Build history of the part. All positions in model axes, mm. A direction names the side the tool comes from. Round coordinates to 2 decimals unless told otherwise and drop trailing zeros. Write each loop counter-clockwise with the first axis right and the second up, starting at its lowest first coordinate (ties: lowest second). Pieces come first, ordered by that corner, then holes. Notation, with made-up numbers: (57, 45.5) -> (103, 45.5) arc R19 cw to (103, 58.5) -> close; hole circle Ø6 at (-3, -17). An arc over 180 degrees is marked (long way). Answer in a Markdown table with one row per item.
Autodesk Inventor part; units mm, degrees
ref_plane "YZ Plane" through (0, 0, 0) normal (1, 0, 0) x (0, 1, 0)
ref_plane "XZ Plane" through (0, 0, 0) normal (0, 1, 0) x (-1, 0, 0)
ref_plane "XY Plane" through (0, 0, 0) normal (0, 0, 1) x (1, 0, 0)
sketch "Skizze1" plane through (0, 0, 0) normal (0, 0, 1) x (1, 0, 0)
  line L0 (0, 0) -> (43.18, 0)
  line L1 (43.18, 0) -> (43.18, 20)
  line L2 (43.18, 20) -> (0, 20)
  line L3 (0, 20) -> (0, 0)
  circle A0 centre (2.54, 2.761) radius 1.651
  circle A1 centre (40.64, 17.239) radius 1.651
  line L4 (21.59, 20) -> (21.59, 0) construction
  line L5 (2.54, 2.761) -> (40.64, 2.761) construction
  line L6 (40.64, 2.761) -> (40.64, 17.239) construction
  line L7 (40.64, 17.239) -> (2.54, 17.239) construction
  line L8 (2.54, 17.239) -> (2.54, 2.761) construction
  line L9 (0, 10) -> (43.18, 10) construction
  line L10 (21.965, 2.2486) -> (21.215, 2.2486)
  line L11 (21.215, 2.2486) -> (21.215, 1.4986)
  line L12 (21.215, 1.4986) -> (21.965, 1.4986)
  line L13 (21.965, 1.4986) -> (21.965, 2.2486)
  line L14 (24.715, 2.2486) -> (23.965, 2.2486)
  line L15 (24.715, 1.4986) -> (24.715, 2.2486)
  line L16 (23.965, 1.4986) -> (24.715, 1.4986)
  line L17 (23.965, 2.2486) -> (23.965, 1.4986)
  line L18 (27.465, 2.2486) -> (26.715, 2.2486)
  line L19 (27.465, 1.4986) -> (27.465, 2.2486)
  line L20 (26.715, 1.4986) -> (27.465, 1.4986)
  line L21 (26.715, 2.2486) -> (26.715, 1.4986)
  line L22 (19.215, 2.2486) -> (18.465, 2.2486)
  line L23 (19.215, 1.4986) -> (19.215, 2.2486)
  line L24 (18.465, 1.4986) -> (19.215, 1.4986)
  line L25 (18.465, 2.2486) -> (18.465, 1.4986)
  line L26 (21.965, 2.2486) -> (21.215, 2.2486)
  line L27 (21.965, 1.4986) -> (21.965, 2.2486)
  line L28 (21.215, 1.4986) -> (21.965, 1.4986)
  line L29 (21.215, 2.2486) -> (21.215, 1.4986)
  line L30 (24.715, 2.2486) -> (23.965, 2.2486)
  line L31 (24.715, 1.4986) -> (24.715, 2.2486)
  line L32 (23.965, 1.4986) -> (24.715, 1.4986)
  line L33 (23.965, 2.2486) -> (23.965, 1.4986)
  line L34 (16.465, 2.2486) -> (15.715, 2.2486)
  line L35 (16.465, 1.4986) -> (16.465, 2.2486)
  line L36 (15.715, 1.4986) -> (16.465, 1.4986)
  line L37 (15.715, 2.2486) -> (15.715, 1.4986)
  line L38 (19.215, 2.2486) -> (18.465, 2.2486)
  line L39 (19.215, 1.4986) -> (19.215, 2.2486)
  line L40 (18.465, 1.4986) -> (19.215, 1.4986)
  line L41 (18.465, 2.2486) -> (18.465, 1.4986)
  line L42 (21.965, 2.2486) -> (21.215, 2.2486)
  line L43 (21.965, 1.4986) -> (21.965, 2.2486)
  line L44 (21.215, 1.4986) -> (21.965, 1.4986)
  line L45 (21.215, 2.2486) -> (21.215, 1.4986)
  point P0 (21.59, 17.239)
  point P1 (40.64, 10)
  point P2 (21.59, 2.2486)
  point P3 (24.34, 2.2486)
  point P4 (27.09, 2.2486)
  point P5 (18.84, 2.2486)
  point P6 (21.59, 2.2486)
  point P7 (24.34, 2.2486)
  point P8 (16.09, 2.2486)
  point P9 (18.84, 2.2486)
  point P10 (21.59, 2.2486)
  dimension "d0" = 43.18
  dimension "d1" = 20
  dimension "d2" = 3.302
  dimension "d4" = 38.1
  dimension "d5" = 14.478
  dimension "d26" = 1.4986
  dimension "d27" = 0.75
  dimension "d30" = 2.75
  dimension "d33" = 2.75
extrude "Extrusion1" add sketch "Skizze1" against normal blind 1.524
sketch "Skizze2" plane through (0, 0, 0) normal (0, 0, 1) x (1, 0, 0)
  circle A0 centre (10.1127, 10) radius 8.128
  circle A1 centre (33.0673, 10) radius 8.128
  line L0 (0, 0) -> (0, 20) construction
  line L1 (0, 10) -> (43.18, 10) construction
  line L2 (43.18, 0) -> (43.18, 20) construction
  line L3 (10.1127, 10) -> (33.0673, 10) construction
  point P0 (21.59, 10)
  dimension "d19" = 16.256
extrude "Extrusion2" add sketch "Skizze2" along normal blind 12.7
fillet "Rundung1" radius 1 2 edges at (24.9393, 10, 12.7) (1.9847, 10, 12.7)
sketch "Skizze3" plane through (0, 0, 0) normal (0, 0, 1) x (1, 0, 0)
  line L0 (43.18, 20) -> (0, 20) construction
  line L1 (21.59, 20) -> (21.59, 16.583) construction
  circle A0 centre (21.59, 16.583) radius 2.286
  point P0 (0, 0)
  dimension "d23" = 4.572
extrude "Extrusion3" add sketch "Skizze3" along normal blind 5.5
properties part number "SRF08"
Q1. Saw through at C-C on z = 4.5. Write the cut outline in (x, y).
A:
| item | result |
|---|---|
| outline | circle Ø16.26 at (10.11, 10); circle Ø4.57 at (21.59, 16.58); circle Ø16.26 at (33.07, 10) |
Q2. Two-plate mould, pull along X, no slides. Class faces 4 (the cylindrical face through (39.33, 16.234, -0.751)), 5 (the flat face through (43.18, 10, -1)), 6 (the flat face through (0, 10, -1)), 7 (the flat face through (10, 10, 12.7)): released by +X, released by -X, zero draft, split by the parting line, or undercut.
A:
| item | result |
|---|---|
| face 4 | undercut |
| face 5 | released by +X |
| face 6 | released by -X |
| face 7 | zero draft |
Q3. Saw through at B-B on z = 11. Write the cut outline in (x, y).
A:
| item | result |
|---|---|
| outline | circle Ø16.26 at (10.11, 10); circle Ø16.26 at (33.07, 10) |
Q4. Saw through at A-A on y = 10. Write the cut outline in (x, z), plus the area to 3 significant figures.
A:
| item | result |
|---|---|
| outline | (0, -1.52) -> (43.18, -1.52) -> (43.18, 0) -> (41.2, 0) -> (41.2, 11.7) arc R1 ccw to (40.2, 12.7) -> (25.94, 12.7) arc R1 ccw to (24.94, 11.7) -> (24.94, 0) -> (18.24, 0) -> (18.24, 11.7) arc R1 ccw to (17.24, 12.7) -> (2.98, 12.7) arc R1 ccw to (1.98, 11.7) -> (1.98, 0) -> (0, 0) -> close |
| area | 478 mm² |
Q5. Wall check: line 1 (Y direction, x = 2.54, z = -1); line 2 (Y direction, x = 40.64, z = -1.1); line 3 (Z direction, x = 30.5, y = 2.25). Give the ranges that are in metal, low to high. Write a range as [from, to].
A:
| item | result |
|---|---|
| line 1 | [0, 1.11], [4.41, 20] |
| line 2 | [0, 15.59], [18.89, 20] |
| line 3 | [-1.52, 0] |
Q6. Which spindle directions (+Z, -Z, +X, -X, +Y, -Y) get a long thin tool onto all of the face, cutting with end or side? Do faces 1 (the flat face through (22, 17, 5.5)), 2 (the cylindrical face through (36.82, 17.21, 5.77)), 3 (the cylindrical face through (1.23, 1.756, -0.751)). Say none if no direction does.
A:
| item | result |
|---|---|
| face 1 | +Z, +Y, -Y |
| face 2 | +Z |
| face 3 | +Z, -Z |
Q7. Drop flat-ended pins along their axis: P1, Ø1, axis at x = 34.5, z = 6, coming from the +Y side; P2, Ø8, axis at y = 8, z = 8.5, coming from the -X side; P3, Ø5, axis at x = 21, y = 16, coming from the +Z side. Give the stop position or say it passes through.
A:
| item | result |
|---|---|
| P1 | y = 18.07 |
| P2 | x = 1.98 |
| P3 | z = 5.5 |
